```python
from build123d import *

# Parameters (mm, degrees)
F0_W     = 82.55
F0_H     = 62.23
F0_W_2   = 73.025
F0_H_2   = 53.975
F1_DEPTH = 50.8
F2_DEPTH = 6.35
F3_R     = 3.96875
F4_DEPTH = 4.1275
F3_W     = 12.7
F3_H     = 9.525
F5_DEPTH = 4.1275


with BuildPart() as f1:
    # F0 (on Top) → F1 (new body)
    with BuildSketch(Plane.XY):
        Rectangle(F0_W, F0_H)
        Rectangle(F0_W_2, F0_H_2, mode=Mode.SUBTRACT)
    extrude(amount=F1_DEPTH)

    # F0 (on Top) → F2 (join)
    with BuildSketch(Plane.XY):
        Rectangle(F0_W_2, F0_H_2)
    extrude(amount=F2_DEPTH)

    # F3 (on face) → F4 (cut, through all)
    with BuildSketch(Plane(origin=(0, 31.115, 0), x_dir=(-1, 0, 0), z_dir=(0, 1, 0))):
        with Locations((-23.491018, 30.719021)):
            Circle(F3_R)
    extrude(amount=-F4_DEPTH, mode=Mode.SUBTRACT)

    # F3 (on face) → F5 (cut, through all)
    with BuildSketch(Plane(origin=(0, 31.115, 0), x_dir=(-1, 0, 0), z_dir=(0, 1, 0))):
        with Locations((7.956224, 31.465962)):
            Rectangle(F3_W, F3_H)
    extrude(amount=-F5_DEPTH, mode=Mode.SUBTRACT)


solid = f1.part
```
Here's how the part is built. I have some questions about the finished solid (model axes, mm). A direction names the side the tool comes from. Give positions to 0.01 mm unless a question says otherwise; leave off trailing zeros. Write each loop counter-clockwise with the first axis right and the second up, starting at its lowest first coordinate (ties: lowest second). Pieces come first, ordered by that corner, then holes. Notation, with made-up numbers: M 78.5,-14.75 L 115.5,-14.75 A22 cw 115.5,5.25 Z; hole C 28.25,79.5 d4. An arc over 180 degrees is marked long. Put each result on its own line as item: value. Start each with the question number.
Item 1: If we section it at A-A, the plane z = 17: Write out the boundary of the cut face in (x, y) (1 decimal).
Item 2: On a 3-axis mill with a long thin cutter (end or side, diameter ignored), from which of +Z, -Z, +X, -X, +Y, -Y can I reach the whole of each face in a straight line? I mean faces 4 (the flat face through (-41.275, 0, 25)), 5 (the flat face through (-1, 26.988, 28)), 6 (the flat face through (-8, 29, 36.228)). Say none if no direction works.
Item 3: I need wall thicknesses on L1, parallel to X at y = 28, z = 30.5 (3 decimals); L2, parallel to Y at x = 22, z = 48 (1 decimal); L3, parallel to X at y = 5, z = 44 (1 decimal). Which ranges of each line are inside material? Lowest first, please. Write a range as from..to.
Item 4: Will this pin go through, and if not, where does the flat tip stop? pin 1 (5 mm diameter, centred on x = -32, y = -7.5, fed in from +Z).
Item 5: Thinking about a two-plate mould opening in Y: for faces 1 (the flat face through (-1, -31.115, 25)), 2 (the flat face through (-14.306, 29, 31)), 3 (the flat face through (-1, 0, 6.35)), which applies, +Y half, -Y half, draft (parallel to the pull), parting line (faces both ways), or undercut?
Values:
1. outline: M -41.3,-31.1 L 41.3,-31.1 L 41.3,31.1 L -41.3,31.1 Z; hole M -36.5,-27 L 36.5,-27 L 36.5,27 L -36.5,27 Z
2. face 4: +Z, -Z, -X, +Y, -Y
2. face 5: +Z
2. face 6: +Y
3. L1: -41.275..-14.306, -1.606..19.528, 27.454..41.275
3. L2: -31.1..-27, 27..31.1
3. L3: -41.3..-36.5, 36.5..41.3
4. pin 1: z = 6.35
5. face 1: -Y half
5. face 2: draft
5. face 3: undercut
